Work out the finished part from the listing and answer in its coordinate system (mm). A direction names the side the tool comes from. Give positions to 0.01 mm unless a question says otherwise; leave off trailing zeros. Loops run counter-clockwise (first coordinate to the right, second up) from the corner with the lowest first, then second, coordinate; pieces in that order, holes last. Notation, with made-up numbers: M 20.5,47 L 61.5,47 A26 ccw 61.5,62 Z; hole C -19,29 d7. An arc over 180 degrees is marked long. Write item = value, one per line. Start each with the question number.
1. Section B-B on z = 7.6 is taken. Determine the outline of the cut face in (x, y) (3 decimals).
2. For faces 1 (the face through (-0.077, 6.678, 2.071)), 2 (the face through (-1.5, 13, 8)), 3 (the face through (-6.005, -27, 2)), 4 (the face through (0, 3.174, 7)), 5 (the face through (0.08, -60.33, 2.07)), determine the directions among +Z, -Z, +X, -X, +Y, -Y from which every point of the face is accessible in a straight line to the end or side of a thin tool.
3. Section D-D on x = 4.25 is taken. Determine the outline of the cut face in (y, z).
4. Section C-C on x = 0 is taken. Determine the outline of the cut face in (y, z), plus the area to 3 significant figures.
5. Consider L1, parallel to Y at x = 0.7, z = 7.6; L2, parallel to Y at x = 0, z = 1.75; L3, parallel to X at y = -9, z = 3.5 (3 decimals). Determine where each line is inside the solid, lowest interval first. Write a range as [from, to].
6. Flat-ended cylindrical pins translate along their axes: pin 1 Ø3.5 at (x, y) = (-0.5, 11.5) entering from -Z; pin 2 Ø3.5 at (y, z) = (11, 7.5) entering from -X; pin 3 Ø2 at (x, y) = (-3, -30.5) entering from +Z. Find the tip coordinate at first contact, or state that the pin passes through.
7. The mould has two halves that part along Y. Classify faces 6 (the face through (3.505, -26, 2)), 7 (the face through (1.5, 13, 8)), 8 (the face through (-0.02, 8.49, 2.71)): released by +Y, released by -Y, zero draft, split by the parting line, or undercut.
8. Section A-A on y = -6.5 is taken. Determine the outline of the cut face in (x, z) (3 decimals).
```python
from build123d import *

# Parameters (mm, degrees)
EXTRUDE_1_DEPTH     = 4.2
EXTRUDE_2_DEPTH     = 5.5
CUT_EXTRUDE_1_DEPTH = 5.5
SKETCH_4_R          = 1.5
CUT_EXTRUDE_2_DEPTH = 10


with BuildPart() as part:
    # 草图1 → 凸台-拉伸1 (new body)
    with BuildSketch(Plane.XY):
        with BuildLine():
            Line((6.005, 3.173780296), (6.005, -56.826219704))
            ThreePointArc((6.005, -56.826219704), (0, -62.831219704), (-6.005, -56.826219704))
            Line((-6.005, -56.826219704), (-6.005, 3.173780296))
            ThreePointArc((-6.005, 3.173780296), (-4.746974036, 6.851587047), (-1.5, 8.988419149))
            Line((-1.5, 8.988419149), (-1.5, 14.988419149))
            Line((-1.5, 14.988419149), (1.5, 14.988419149))
            Line((1.5, 14.988419149), (1.5, 8.988419149))
            ThreePointArc((1.5, 8.988419149), (4.746974036, 6.851587047), (6.005, 3.173780296))
        make_face()
        with BuildLine():
            Line((3.505, 3.173780296), (3.505, -56.826219704))
            ThreePointArc((3.505, -56.826219704), (0, -60.331219704), (-3.505, -56.826219704))
            Line((-3.505, -56.826219704), (-3.505, 3.173780296))
            ThreePointArc((-3.505, 3.173780296), (0, 6.678780296), (3.505, 3.173780296))
        make_face(mode=Mode.SUBTRACT)
    extrude(amount=EXTRUDE_1_DEPTH)

    # 草图2 → 凸台-拉伸2 (add)
    with BuildSketch(Plane.XY.offset(4.2)):
        with BuildLine():
            Line((1.5, 14.988419149), (-1.5, 14.988419149))
            Line((-1.5, 14.988419149), (-1.5, 8.988419149))
            ThreePointArc((-1.5, 8.988419149), (-4.746974036, 6.851587047), (-6.005, 3.173780296))
            Line((-6.005, 3.173780296), (6.005, 3.173780296))
            ThreePointArc((6.005, 3.173780296), (4.746974036, 6.851587047), (1.5, 8.988419149))
            Line((1.5, 8.988419149), (1.5, 14.988419149))
        make_face()
    extrude(amount=EXTRUDE_2_DEPTH)

    # 草图3 → 切除-拉伸1 (cut)
    with BuildSketch(Plane(origin=(0, 0, 0), x_dir=(-1, 0, 0), z_dir=(0, 0, -1))):
        with BuildLine():
            Line((-1.5, 14.988419149), (1.5, 14.988419149))
            Line((1.5, 14.988419149), (1.5, 8.988419149))
            ThreePointArc((1.5, 8.988419149), (0, 8.488419149), (-1.5, 8.988419149))
            Line((-1.5, 8.988419149), (-1.5, 14.988419149))
        make_face()
    extrude(amount=-CUT_EXTRUDE_1_DEPTH, mode=Mode.SUBTRACT)

    # 草图4 → 切除-拉伸2 (cut)
    with BuildSketch(Plane(origin=(1.5, 0, 0), x_dir=(0, 0, -1), z_dir=(1, 0, 0))):
        with Locations((-7.6, 10.988419149)):
            Circle(SKETCH_4_R)
    extrude(amount=-CUT_EXTRUDE_2_DEPTH, mode=Mode.SUBTRACT)


solid = part.part
```
Verdict:
q1.outline = M -6.005,3.174 L 6.005,3.174 A6.005 ccw 1.5,8.988 L 1.5,9.488 L -1.5,9.488 L -1.5,8.988 A6.005 ccw Z; M -1.5,12.488 L 1.5,12.488 L 1.5,14.988 L -1.5,14.988 Z
q2.face_1 = -Z
q2.face_2 = +Z, -Z, -X, +Y
q2.face_3 = +Z, -Z, -X, +Y, -Y
q2.face_4 = +Z, +X, -X, -Y
q2.face_5 = +Z, -Z
q3.outline = M -61.07,0 L 7.42,0 L 7.42,9.7 L 3.17,9.7 L 3.17,4.2 L -61.07,4.2 Z
q4.outline = M -62.83,0 L -60.33,0 L -60.33,4.2 L -62.83,4.2 Z; M 3.17,4.2 L 6.68,4.2 L 6.68,0 L 8.49,0 L 8.49,5.5 L 14.99,5.5 L 14.99,9.7 L 3.17,9.7 Z; hole C 10.99,7.6 d3
q4.area = 67.6 mm2
q5.L1 = [3.17, 9.49], [12.49, 14.99]
q5.L2 = [-62.83, -60.33], [6.68, 8.49]
q5.L3 = [-6.005, -3.505], [3.505, 6.005]
q6.pin_1 = 5.5
q6.pin_2 = -1.5
q6.pin_3 = 4.2
q7.face_6 = undercut
q7.face_7 = zero draft
q7.face_8 = released by +Y
q8.outline = M -6.005,0 L -3.505,0 L -3.505,4.2 L -6.005,4.2 Z; M 3.505,0 L 6.005,0 L 6.005,4.2 L 3.505,4.2 Z
